Part model, mm, in its own coordinate system. Face numbers are marked on the shaded views. Round coordinates to 2 decimals unless told otherwise and drop trailing zeros. Write each loop counter-clockwise with the first axis right and the second up, starting at its lowest first coordinate (ties: lowest second). Pieces come first, ordered by that corner, then holes. Notation, with made-up numbers: M 34.5,9.5 L 39.5,9.5 A14 ccw 39.5,30.5 Z; hole C 1.25,7.25 d4. An arc over 180 degrees is marked long. Use one line per item in the form item = value. Start each with the question number.
Item 1: Flat gauge pins, fed straight in: pin 1 Ø3 at (x, z) = (54.5, -4.5) entering from -Y; pin 2 Ø4 at (x, y) = (139.5, -70.5) entering from -Z; pin 3 Ø13 at (x, z) = (102.5, -29.5) entering from -Y. Where does each tip first touch, or does it go through?
Item 2: Cut at C-C, the plane y = -29.5. Give the cut face in (x, z).
Item 3: Probe L1, parallel to Y at x = 79, z = -8; L2, parallel to Y at x = 56, z = -23.5; L3, parallel to Y at x = 118, z = -31.5. List the from-to ranges inside material, lowest first.
Item 4: Mould opens along Y. For the marked faces 1 and 2 say: +Y half, -Y half, draft (parallel to the pull), parting line (faces both ways), or undercut.
Item 5: Cut at A-A, the plane z = -27.5. Give the cut face in (x, y), then the cut area to 3 significant figures.
Item 6: Cut at B-B, the plane z = -7. Give the cut face in (x, y), then the cut area to 3 significant figures.
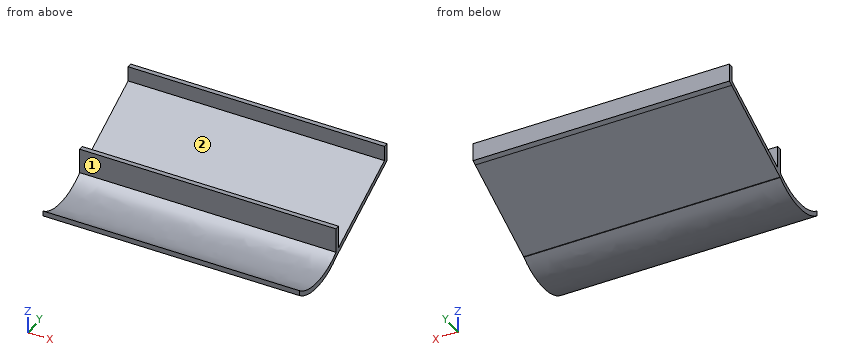
from build123d import *

# Parameters (mm, degrees)
EXTRUDE_1_DEPTH = 163.8


with BuildPart() as part:
    # 草图1 → 凸台-拉伸1 (new body)
    with BuildSketch(Plane(origin=(0, 0, 0), x_dir=(0, 0, -1), z_dir=(1, 0, 0))):
        with BuildLine():
            Line((9.7, 0), (36.35874095, -53.63))
            Line((36.35874095, -53.63), (21.85, -53.63))
            Line((21.85, -53.63), (21.85, -56.63))
            Line((21.85, -56.63), (37.85, -56.63))
            add(Edge.make_bspline(
                [(37.85, -56.63), (46.953982553, -69.060712167), (47.499791502, -87.422152902), (37.85, -99.63)],
                knots=[0, 0, 0, 0, 1, 1, 1, 1], degree=3))
            Line((37.85, -99.63), (41.200202017, -99.63))
            add(Edge.make_bspline(
                [(41.200202017, -56.63), (50.30418457, -69.060712167), (50.849993519, -87.422152902), (41.200202017, -99.63)],
                knots=[0, 0, 0, 0, 1, 1, 1, 1], degree=3))
            Line((41.200202017, -56.63), (41.042940367, -56.313633136))
            Line((41.042940367, -56.313633136), (12.892940367, 0.316366864))
            Line((12.892940367, 0.316366864), (11.558942967, 3))
            Line((11.558942967, 3), (0, 3))
            Line((0, 3), (0, 0))
            Line((0, 0), (9.7, 0))
        make_face()
    extrude(amount=EXTRUDE_1_DEPTH)


solid = part.part
Model answer:
q1.pin_1 = 0
q1.pin_2 = -47.75
q1.pin_3 = -56.63
q2.outline = M 0,-27.71 L 163.8,-27.71 L 163.8,-24.36 L 0,-24.36 Z
q3.L1 = 0 to 3
q3.L2 = -56.63 to -53.63, -27.76 to -21.02
q3.L3 = -56.63 to -53.63, -43.86 to -37.12
q4.face_1 = -Y half
q4.face_2 = undercut
q5.outline = M 0,-56.63 L 163.8,-56.63 L 163.8,-53.63 L 0,-53.63 Z; M 0,-35.81 L 163.8,-35.81 L 163.8,-29.07 L 0,-29.07 Z
q5.area = 1,600 mm²
q6.outline = M 0,0 L 163.8,0 L 163.8,3 L 0,3 Z
q6.area = 491 mm²
